Input: dimensioned drawing with shaded views. Units: mm. Origin: part minimum x, y, z. Coordinates: 2 decimals unless noted, no trailing zeros. Write each loop counter-clockwise with the first axis right and the second up, starting at its lowest first coordinate (ties: lowest second). Pieces come first, ordered by that corner, then holes. Notation, with made-up numbers: (82, -14.75) -> (141, -14.75) arc R16 cw to (141, 1.25) -> close; hole circle Ø5 at (19, 38.25). An arc over 180 degrees is marked (long way). One line per item, written item: value. Start each with the question number.
1. Section query A-A, the plane y = 15. Output: boundary loops of the cut face in (x, z) (3 decimals).
2. Section query D-D, the plane z = 2.9. Output: boundary loops of the cut face in (x, y) (3 decimals).
3. Section query B-B, the plane x = 27.8. Output: boundary loops of the cut face in (y, z) (3 decimals), and give its area (3 significant figures).
4. Mould query, pull axis X, two halves, no side actions, for the marked faces 1 and 2. Classes: released by +X, released by -X, zero draft, split by the parting line, or undercut.
5. Section query C-C, the plane x = 35. Output: boundary loops of the cut face in (y, z), and give its area (3 significant figures).
6. Line query: line 1 (Y direction, x = 27.8, z = 3.55) (3 decimals); line 2 (X direction, y = 14.5, z = 3.7); line 3 (X direction, y = 39, z = 4.1). Output: solid intervals per line, ascending.
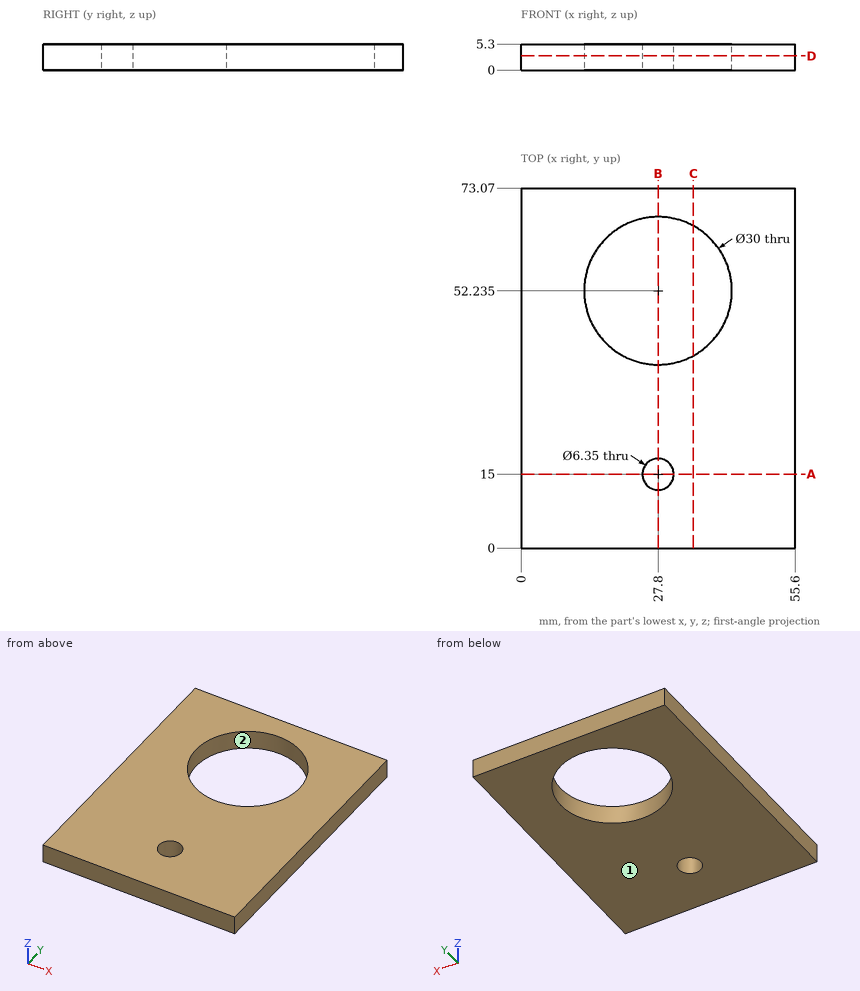
Computed values:
1. outline: (0, 0) -> (24.625, 0) -> (24.625, 5.3) -> (0, 5.3) -> close; (30.975, 0) -> (55.6, 0) -> (55.6, 5.3) -> (30.975, 5.3) -> close
2. outline: (0, 0) -> (55.6, 0) -> (55.6, 73.07) -> (0, 73.07) -> close; hole circle Ø30 at (27.8, 52.235); hole circle Ø6.35 at (27.8, 15)
3. outline: (0, 0) -> (11.825, 0) -> (11.825, 5.3) -> (0, 5.3) -> close; (18.175, 0) -> (37.235, 0) -> (37.235, 5.3) -> (18.175, 5.3) -> close; (67.235, 0) -> (73.07, 0) -> (73.07, 5.3) -> (67.235, 5.3) -> close
3. area: 195 mm²
4. face 1: zero draft
4. face 2: undercut
5. outline: (0, 0) -> (39.08, 0) -> (39.08, 5.3) -> (0, 5.3) -> close; (65.39, 0) -> (73.07, 0) -> (73.07, 5.3) -> (65.39, 5.3) -> close
5. area: 248 mm²
6. line 1: y = 0 to 11.825, 18.175 to 37.235, 67.235 to 73.07
6. line 2: x = 0 to 24.66, 30.94 to 55.6
6. line 3: x = 0 to 20.74, 34.86 to 55.6
